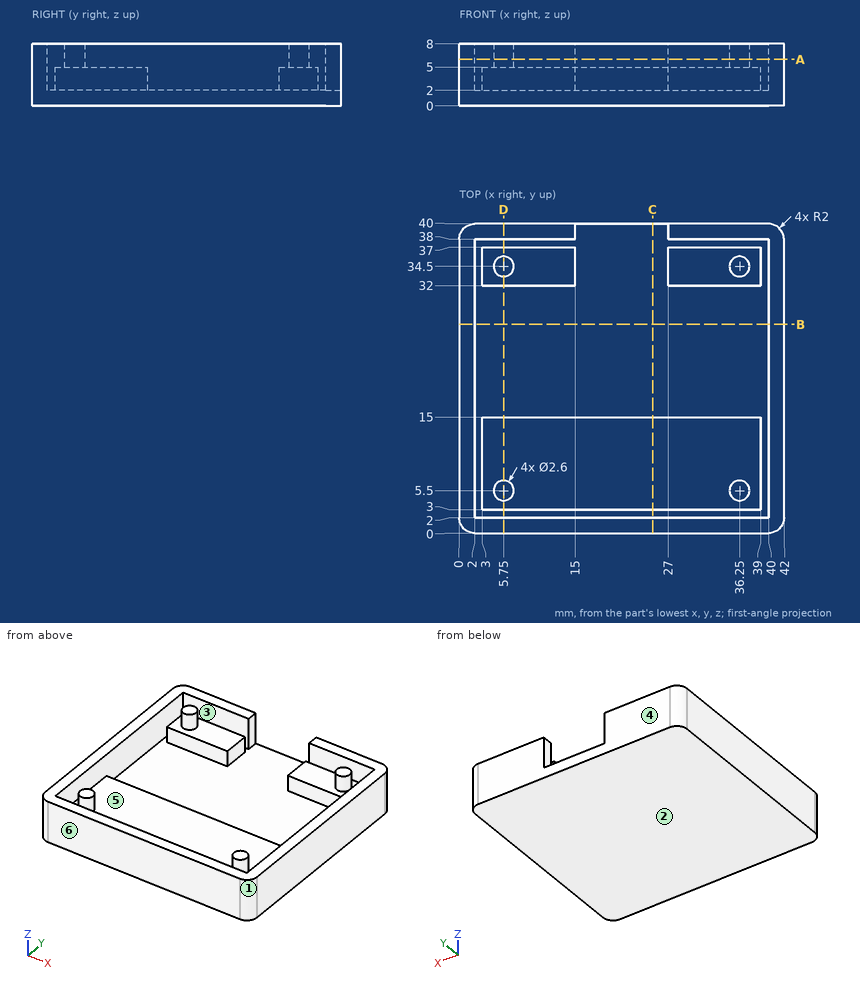
The drawing under review shows one solid part. Ordinate dimensions are in mm from its lowest x, y, z. A direction names the side the tool comes from. Coordinates: 2 decimals unless noted, no trailing zeros. Write each loop counter-clockwise with the first axis right and the second up, starting at its lowest first coordinate (ties: lowest second). Pieces come first, ordered by that corner, then holes. Notation, with made-up numbers: (-36.75, 28) -> (-6.75, 28) arc R32 cw to (-6.75, 64) -> close; hole circle Ø2 at (35, 37). An arc over 180 degrees is marked (long way). Write each question's results on one line, items separated by ' | '. Start each with the question number.
1) Wall thickness on L1, parallel to X at y = 36, z = 4.25; L2, parallel to X at y = 3.5, z = 4.75; L3, parallel to Y at x = 27.5, z = 2.5: over which ranges is each line inside the solid? List them lowest first. Write a range as [from, to].
2) Consider section A-A (z = 6). Write out the cut boundary in (x, y).
3) Consider section D-D (x = 5.75). Write out the cut boundary in (y, z).
4) Consider section C-C (x = 25). Write out the cut boundary in (y, z).
5) Consider section B-B (y = 27). Write out the cut boundary in (x, z).
6) The part is to be moulded in two halves that separate along Y. For the marked faces 1, 2, 3 and 4, say which applies: +Y half, -Y half, draft (parallel to the pull), parting line (faces both ways), or undercut.
7) For the marked faces 5 and 6, list the 3-axis set-ups (+Z, -Z, +X, -X, +Y, -Y) from which the entire face can be reached by the end or side of a thin tool; tool diameter is ignored.
8) Insertion check: pin 1 (3 mm diameter, centred on y = 21.5, z = 6, fed in from -X); pin 2 (1.5 mm diameter, centred on x = 24.5, z = 3.5, fed in from +Y); pin 3 (1.5 mm diameter, centred on x = 5.5, y = 9, fed in from +Z). Each pin has a flat end and moves straight along its axis. Give the tip position at first contact, or say it passes through.
Geometry says:
1) L1: [0, 2], [3, 15], [27, 39], [40, 42] | L2: [0, 2], [3, 39], [40, 42] | L3: [0, 2], [3, 15], [32, 37], [38, 40]
2) outline: (0, 2) arc R2 ccw to (2, 0) -> (40, 0) arc R2 ccw to (42, 2) -> (42, 38) arc R2 ccw to (40, 40) -> (27, 40) -> (27, 38) -> (40, 38) -> (40, 2) -> (2, 2) -> (2, 38) -> (15, 38) -> (15, 40) -> (2, 40) arc R2 ccw to (0, 38) -> close; circle Ø2.6 at (5.75, 5.5); circle Ø2.6 at (5.75, 34.5); circle Ø2.6 at (36.25, 5.5); circle Ø2.6 at (36.25, 34.5)
3) outline: (0, 0) -> (40, 0) -> (40, 8) -> (38, 8) -> (38, 2) -> (37, 2) -> (37, 5) -> (35.8, 5) -> (35.8, 8) -> (33.2, 8) -> (33.2, 5) -> (32, 5) -> (32, 2) -> (15, 2) -> (15, 5) -> (6.8, 5) -> (6.8, 8) -> (4.2, 8) -> (4.2, 5) -> (3, 5) -> (3, 2) -> (2, 2) -> (2, 8) -> (0, 8) -> close
4) outline: (0, 0) -> (40, 0) -> (40, 2) -> (15, 2) -> (15, 5) -> (3, 5) -> (3, 2) -> (2, 2) -> (2, 8) -> (0, 8) -> close
5) outline: (0, 0) -> (42, 0) -> (42, 8) -> (40, 8) -> (40, 2) -> (2, 2) -> (2, 8) -> (0, 8) -> close
6) face 1: -Y half | face 2: draft | face 3: undercut | face 4: +Y half
7) face 5: +Z | face 6: +Z, -Z, +X, -X, -Y
8) pin 1: x = 0 | pin 2: y = 15 | pin 3: z = 5
